Geometry: final body of the model. Coordinates: model frame, mm. A direction names the side the tool comes from. Round coordinates to 2 decimals unless told otherwise and drop trailing zeros. Write item = value, one per line. Start each with the question number.
Item 1: Line query: line 1 (Z direction, x = -17, y = -337); line 2 (Z direction, x = -16, y = -206.5); line 3 (X direction, y = -179, z = 2.5). Output: solid intervals per line, ascending. Write a range as from..to.
Item 2: Section A-A (y = -299.5). Count the separate pieces of the cut face and the enclosed holes in it, plus the area to 3 significant figures.
Item 3: Draft query along Z for faces 1 (the flat face through (20.5, -177, 10)), 2 (the flat face through (9, -177, -19)), 3 (the flat face through (0, -177, 10)). Return one class per face: pulls with the +Z half, pulls with the -Z half, needs draft (parallel to the pull), parting line crosses it, or undercut.
Item 4: Access query for faces 4 (the flat face through (0, -177, -10)), 5 (the flat face through (-20.5, -177, 11)). Directions: +Z, -Z, +X, -X, +Y, -Y. A direction counts if a zero-diameter tool reaches every point of the face in a straight line with its end or side. Return the directions, or none.
from build123d import *

# Parameters (mm, degrees)
F1_DEPTH = 360
F3_D     = 4.2
F4_R     = 2
F5_R     = 2
F6_R     = 2
F7_R     = 2
F8_R     = 2
F9_R     = 2


with BuildPart() as f1:
    # F0 (on Front) → F1 (new body)
    with BuildSketch(Plane.XZ):
        Polygon((0, -10), (0, 0), (0, 10), (-7.5, 10), (-7.5, 17), (-3.5, 17), (-3.5, 19), (-20.5, 19), (-20.5, 2), (-18.5, 2), (-18.5, 6), (-11.5, 6), (-11.5, 0), (-11.5, -6), (-18.5, -6), (-18.5, -2), (-20.5, -2), (-20.5, -19), (-3.5, -19), (-3.5, -17), (-7.5, -17), (-7.5, -10), align=None)
        Polygon((0, 10), (0, 0), (0, -10), (7.5, -10), (7.5, -17), (3.5, -17), (3.5, -19), (20.5, -19), (20.5, -2), (18.5, -2), (18.5, -6), (11.5, -6), (11.5, 0), (11.5, 6), (18.5, 6), (18.5, 2), (20.5, 2), (20.5, 19), (3.5, 19), (3.5, 17), (7.5, 17), (7.5, 10), align=None)
    extrude(amount=F1_DEPTH)

    # F3 (through all)
    with Locations(Plane.XZ.offset(360)):
        with Locations((15.5, 15), (-16.5, 15), (15.5, -17), (-16.5, -17)):
            Hole(F3_D / 2)

    # F4
    f4_edges = [f1.edges().sort_by_distance(p)[0] for p in [
        (-7.5, -180, 10),
        (-18.5, -180, -6),
        (-7.5, -180, -17),
        (11.5, -180, -6),
    ]]
    fillet(f4_edges, radius=F4_R)

    # F5
    f5_edges = [f1.edges().sort_by_distance(p)[0] for p in [
        (7.5, -180, 10),
    ]]
    fillet(f5_edges, radius=F5_R)

    # F6
    f6_edges = [f1.edges().sort_by_distance(p)[0] for p in [
        (-11.5, -180, -6),
        (7.5, -180, -10),
        (18.5, -180, 6),
    ]]
    fillet(f6_edges, radius=F6_R)

    # F7
    f7_edges = [f1.edges().sort_by_distance(p)[0] for p in [
        (7.5, -180, -17),
        (18.5, -180, -6),
    ]]
    fillet(f7_edges, radius=F7_R)

    # F8
    f8_edges = [f1.edges().sort_by_distance(p)[0] for p in [
        (-7.5, -180, -10),
        (-18.5, -180, 6),
        (-7.5, -180, 17),
        (11.5, -180, 6),
    ]]
    fillet(f8_edges, radius=F8_R)

    # F9
    f9_edges = [f1.edges().sort_by_distance(p)[0] for p in [
        (-11.5, -180, 6),
        (7.5, -180, 17),
    ]]
    fillet(f9_edges, radius=F9_R)


solid = f1.part
Taken from the geometry:
q1.line_1 = -14.96..-5.94, 5.94..12.96, 17.04..19
q1.line_2 = -14.96..-6, 6..12.96, 17.04..19
q1.line_3 = -20.5..-18.5, -11.5..11.5, 18.5..20.5
q2.separate_pieces = 1
q2.enclosed_holes = 2
q2.area = 1,090 mm^2
q3.face_1 = needs draft
q3.face_2 = pulls with the -Z half
q3.face_3 = undercut
q4.face_4 = +Y, -Y
q4.face_5 = +Z, -Z, -X, +Y, -Y
